Verification items for the finished model (mm, model axes). A direction names the side the tool comes from. Give positions to 0.01 mm unless a question says otherwise; leave off trailing zeros. Write each loop counter-clockwise with the first axis right and the second up, starting at its lowest first coordinate (ties: lowest second). Pieces come first, ordered by that corner, then holes. Notation, with made-up numbers: M 51,-25 L 99,-25 A5 cw 99,-18 Z; hole C 42.5,42 d4. An arc over 180 degrees is marked long. Write item = value, one per line.
from build123d import *

# Parameters (mm, degrees)
F0_W     = 220
F0_H     = 140
F0_W_2   = 200
F0_H_2   = 115
F1_DEPTH = 2
F2_DEPTH = 5
F3_DEPTH = 10


with BuildPart() as f1:
    # F0 (on Top) → F1 (new body)
    with BuildSketch(Plane.XY):
        with Locations((-1.9406005144, 8.4791064262)):
            Rectangle(F0_W, F0_H)
        Polygon((106.0593994856, 76.4791064262), (106.0593994856, 71.4791064262), (107.0593994856, 71.4791064262), (107.0593994856, 69.4791064262), (107.0593994856, 54.4791064262), (106.0593994856, 54.4791064262), (106.0593994856, -42.5208935738), (107.0593994856, -42.5208935738), (107.0593994856, -57.5208935738), (107.0593994856, -59.5208935738), (106.0593994856, -59.5208935738), (105.0593994856, -59.5208935738), (90.0593994856, -59.5208935738), (-91.9406005144, -59.5208935738), (-106.9406005144, -59.5208935738), (-108.9406005144, -59.5208935738), (-109.9406005144, -59.5208935738), (-109.9406005144, 76.4791064262), align=None, mode=Mode.SUBTRACT)
        Polygon((90.0593994856, 69.4791064262), (90.0593994856, 71.4791064262), (105.0593994856, 71.4791064262), (106.0593994856, 71.4791064262), (106.0593994856, 76.4791064262), (-109.9406005144, 76.4791064262), (-109.9406005144, -59.5208935738), (-108.9406005144, -59.5208935738), (-108.9406005144, -57.5208935738), (-108.9406005144, -42.5208935738), (-106.9406005144, -42.5208935738), (-106.9406005144, -57.5208935738), (-91.9406005144, -57.5208935738), (-91.9406005144, -59.5208935738), (90.0593994856, -59.5208935738), (90.0593994856, -57.5208935738), (105.0593994856, -57.5208935738), (105.0593994856, -42.5208935738), (106.0593994856, -42.5208935738), (106.0593994856, 54.4791064262), (105.0593994856, 54.4791064262), (105.0593994856, 69.4791064262), align=None)
        Polygon((-106.9406005144, 54.4791064262), (-108.9406005144, 54.4791064262), (-108.9406005144, 69.4791064262), (-108.9406005144, 71.4791064262), (-106.9406005144, 71.4791064262), (-91.9406005144, 71.4791064262), (-91.9406005144, 69.4791064262), (-106.9406005144, 69.4791064262), align=None, mode=Mode.SUBTRACT)
        with Locations((-1.9406005144, 8.9791064262)):
            Rectangle(F0_W_2, F0_H_2, mode=Mode.SUBTRACT)
        Polygon((-108.9406005144, -57.5208935738), (-108.9406005144, -59.5208935738), (-106.9406005144, -59.5208935738), (-91.9406005144, -59.5208935738), (-91.9406005144, -57.5208935738), (-106.9406005144, -57.5208935738), (-106.9406005144, -42.5208935738), (-108.9406005144, -42.5208935738), align=None)
        Polygon((-108.9406005144, 69.4791064262), (-108.9406005144, 54.4791064262), (-106.9406005144, 54.4791064262), (-106.9406005144, 69.4791064262), (-91.9406005144, 69.4791064262), (-91.9406005144, 71.4791064262), (-106.9406005144, 71.4791064262), (-108.9406005144, 71.4791064262), align=None)
        Polygon((105.0593994856, 71.4791064262), (90.0593994856, 71.4791064262), (90.0593994856, 69.4791064262), (105.0593994856, 69.4791064262), (105.0593994856, 54.4791064262), (106.0593994856, 54.4791064262), (106.0593994856, 71.4791064262), align=None)
        Polygon((106.0593994856, -59.5208935738), (106.0593994856, -42.5208935738), (105.0593994856, -42.5208935738), (105.0593994856, -57.5208935738), (90.0593994856, -57.5208935738), (90.0593994856, -59.5208935738), (105.0593994856, -59.5208935738), align=None)
        Polygon((107.0593994856, 71.4791064262), (106.0593994856, 71.4791064262), (106.0593994856, 54.4791064262), (107.0593994856, 54.4791064262), (107.0593994856, 69.4791064262), align=None)
        Polygon((107.0593994856, -42.5208935738), (106.0593994856, -42.5208935738), (106.0593994856, -59.5208935738), (107.0593994856, -59.5208935738), (107.0593994856, -57.5208935738), align=None)
    extrude(amount=-F1_DEPTH)

    # F0 (on Top) → F2 (join)
    with BuildSketch(Plane.XY):
        Polygon((-108.9406005144, 69.4791064262), (-108.9406005144, 54.4791064262), (-106.9406005144, 54.4791064262), (-106.9406005144, 69.4791064262), (-91.9406005144, 69.4791064262), (-91.9406005144, 71.4791064262), (-106.9406005144, 71.4791064262), (-108.9406005144, 71.4791064262), align=None)
        Polygon((-108.9406005144, -57.5208935738), (-108.9406005144, -59.5208935738), (-106.9406005144, -59.5208935738), (-91.9406005144, -59.5208935738), (-91.9406005144, -57.5208935738), (-106.9406005144, -57.5208935738), (-106.9406005144, -42.5208935738), (-108.9406005144, -42.5208935738), align=None)
        Polygon((105.0593994856, 71.4791064262), (90.0593994856, 71.4791064262), (90.0593994856, 69.4791064262), (105.0593994856, 69.4791064262), (105.0593994856, 54.4791064262), (106.0593994856, 54.4791064262), (106.0593994856, 71.4791064262), align=None)
        Polygon((106.0593994856, -59.5208935738), (106.0593994856, -42.5208935738), (105.0593994856, -42.5208935738), (105.0593994856, -57.5208935738), (90.0593994856, -57.5208935738), (90.0593994856, -59.5208935738), (105.0593994856, -59.5208935738), align=None)
    extrude(amount=F2_DEPTH)

    # F0 (on Top) → F3 (join)
    with BuildSketch(Plane.XY):
        with Locations((-1.9406005144, 8.4791064262)):
            Rectangle(F0_W, F0_H)
        Polygon((106.0593994856, 76.4791064262), (106.0593994856, 71.4791064262), (107.0593994856, 71.4791064262), (107.0593994856, 69.4791064262), (107.0593994856, 54.4791064262), (106.0593994856, 54.4791064262), (106.0593994856, -42.5208935738), (107.0593994856, -42.5208935738), (107.0593994856, -57.5208935738), (107.0593994856, -59.5208935738), (106.0593994856, -59.5208935738), (105.0593994856, -59.5208935738), (90.0593994856, -59.5208935738), (-91.9406005144, -59.5208935738), (-106.9406005144, -59.5208935738), (-108.9406005144, -59.5208935738), (-109.9406005144, -59.5208935738), (-109.9406005144, 76.4791064262), align=None, mode=Mode.SUBTRACT)
        Polygon((107.0593994856, -42.5208935738), (106.0593994856, -42.5208935738), (106.0593994856, -59.5208935738), (107.0593994856, -59.5208935738), (107.0593994856, -57.5208935738), align=None)
        Polygon((107.0593994856, 71.4791064262), (106.0593994856, 71.4791064262), (106.0593994856, 54.4791064262), (107.0593994856, 54.4791064262), (107.0593994856, 69.4791064262), align=None)
    extrude(amount=F3_DEPTH)


solid = f1.part
1) Tool access check on faces 1 (the flat face through (-111.941, 7, 4)), 2 (the flat face through (-104, -58, 5)). Record the directions out of +Z, -Z, +X, -X, +Y, -Y that give a thin tool (end or side, any length) a straight path to the whole face; none if there is none.
From the geometry:
face_1 = +Z, -Z, -X, +Y, -Y
face_2 = +Z
2) Material ranges on probe 1 along X at (y, z) = (60.5, 3.75); probe 2 along X at (y, z) = (35, 0.5); probe 3 along X at (y, z) = (14.5, -0.75), recorded low to high. Write a range as from..to.
From the geometry:
probe_1 = -111.94..-109.94, -108.94..-106.94, 105.06..108.06
probe_2 = -111.94..-109.94, 106.06..108.06
probe_3 = -111.94..-101.94, 98.06..108.06
3) Cross-section at D-D on y = 64. Record the boundary of the cut face in (x, z), plus the area to 3 significant figures.
From the geometry:
outline = M -111.94,-2 L -101.94,-2 L -101.94,0 L -106.94,0 L -106.94,5 L -108.94,5 L -108.94,0 L -109.94,0 L -109.94,10 L -111.94,10 Z; M 98.06,-2 L 108.06,-2 L 108.06,10 L 106.06,10 L 106.06,5 L 105.06,5 L 105.06,0 L 98.06,0 Z
area = 95.0 mm^2
4) Cross-section at C-C on z = 8. Record the boundary of the cut face in (x, y), plus the area to 3 significant figures.
From the geometry:
outline = M -111.94,-61.52 L 108.06,-61.52 L 108.06,78.48 L -111.94,78.48 Z; hole M -109.94,-59.52 L 106.06,-59.52 L 106.06,76.48 L -109.94,76.48 Z
area = 1,420 mm^2
5) Draft check along Y on faces 3 (the flat face through (-11, -53, -2)), 4 (the flat face through (97, 69.479, 2)). Enter one of: +Y half, -Y half, draft (parallel to the pull), parting line (faces both ways), or undercut.
From the geometry:
face_3 = draft
face_4 = undercut
6) Cross-section at B-B on x = 70. Record the boundary of the cut face in (y, z), plus the area to 3 significant figures.
From the geometry:
outline = M -61.52,-2 L -48.52,-2 L -48.52,0 L -59.52,0 L -59.52,10 L -61.52,10 Z; M 66.48,-2 L 78.48,-2 L 78.48,10 L 76.48,10 L 76.48,0 L 66.48,0 Z
area = 90.0 mm^2
7) Cross-section at A-A on y = 43. Record the boundary of the cut face in (x, z), plus the area to 3 significant figures.
From the geometry:
outline = M -111.94,-2 L -101.94,-2 L -101.94,0 L -109.94,0 L -109.94,10 L -111.94,10 Z; M 98.06,-2 L 108.06,-2 L 108.06,10 L 106.06,10 L 106.06,0 L 98.06,0 Z
area = 80.0 mm^2
